Verification items for the finished model (mm, model axes). Face numbers are marked on the shaded views. A direction names the side the tool comes from. Coordinates: 2 decimals unless noted, no trailing zeros. Order: outer loops, then holes, each group sorted by start corner. A loop starts at its lowest first (then second) coordinate and runs counter-clockwise, first axis right, second up. Notation, with made-up numbers: (70.5, 7) -> (78.5, 7) arc R34 cw to (78.5, 42) -> close; hole circle Ø7 at (19, -37.75). An arc over 180 degrees is marked (long way). Answer as CSV lines item,"result".
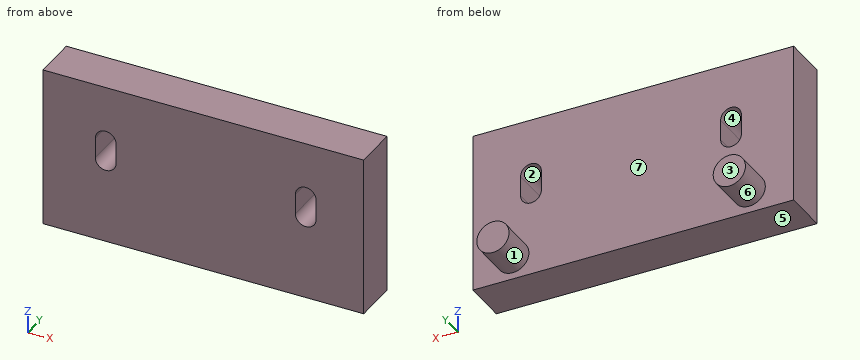
```python
from build123d import *

# Parameters (mm, degrees)
SKETCH1_W           = 301.378206246
SKETCH1_H           = 151.435088782
BOSS_EXTRUDE1_DEPTH = 41.656
CUT_EXTRUDE1_DEPTH  = 214.376
SKETCH3_R           = 15.161110792
BOSS_EXTRUDE2_DEPTH = 35.56


with BuildPart() as part:
    # Sketch1 → Boss-Extrude1 (new body)
    with BuildSketch(Plane(origin=(0, 0, 0), x_dir=(1, 0, 0), z_dir=(0, 1, 0))):
        with Locations((-2.237956977, 0)):
            Rectangle(SKETCH1_W, SKETCH1_H)
    extrude(amount=BOSS_EXTRUDE1_DEPTH)

    # Sketch2 → Cut-Extrude1 (cut)
    with BuildSketch(Plane(origin=(0, 41.656, 0), x_dir=(1, 0, 0), z_dir=(0, 1, 0))):
        with BuildLine():
            Line((-103.753069352, -3.904427399), (-103.753069352, -22.938510969))
            ThreePointArc((-103.753069352, -22.938510969), (-93.992000854, -32.699579467), (-84.230932357, -22.938510969))
            Line((-84.230932357, -22.938510969), (-84.230932357, -3.904427399))
            ThreePointArc((-84.230932357, -3.904427399), (-93.992000854, 5.856641099), (-103.753069352, -3.904427399))
        make_face()
    cut_extrude1 = extrude(amount=-CUT_EXTRUDE1_DEPTH, mode=Mode.SUBTRACT)

    # Sketch3 → Boss-Extrude2 (add)
    with BuildSketch(Plane(origin=(0, 41.656, 0), x_dir=(1, 0, 0), z_dir=(0, 1, 0))):
        with Locations(Location((-111.073870725, 54.487556638, 0), (0, 0, 270))):
            Circle(SKETCH3_R)
    boss_extrude2 = extrude(amount=BOSS_EXTRUDE2_DEPTH)

    # Mirror1: Cut-Extrude1, Boss-Extrude2 across plane
    add(cut_extrude1.mirror(Plane(origin=(0, 0, 0), x_dir=(0, 0, 1), z_dir=(1, 0, 0))), mode=Mode.SUBTRACT)
    add(boss_extrude2.mirror(Plane(origin=(0, 0, 0), x_dir=(0, 0, 1), z_dir=(1, 0, 0))))


solid = part.part
```
Item 1: Section check C-C, the plane x = -118. Record the boundary of the cut face in (y, z), plus the area to 3 significant figures.
Answer list:
outline,"(0, -75.72) -> (41.66, -75.72) -> (41.66, -67.97) -> (77.22, -67.97) -> (77.22, -41) -> (41.66, -41) -> (41.66, 75.72) -> (0, 75.72) -> close"
area,"7,270 mm2"
Item 2: Section check A-A, the plane y = 27. Record the boundary of the cut face in (x, z).
Answer list:
outline,"(-152.93, -75.72) -> (148.45, -75.72) -> (148.45, 75.72) -> (-152.93, 75.72) -> close; hole (-103.75, 3.9) arc R9.76 ccw to (-84.23, 3.9) -> (-84.23, 22.94) arc R9.76 ccw to (-103.75, 22.94) -> close; hole (84.23, 3.9) arc R9.76 ccw to (103.75, 3.9) -> (103.75, 22.94) arc R9.76 ccw to (84.23, 22.94) -> close"
Item 3: Tool access check on the marked faces 1, 2 and 3. Record the directions out of +Z, -Z, +X, -X, +Y, -Y that give a thin tool (end or side, any length) a straight path to the whole face; none if there is none.
Answer list:
face 1,"+Y"
face 2,"+Y, -Y"
face 3,"+Z, -Z, +X, -X, +Y"
Item 4: Section check B-B, the plane y = 60. Record the boundary of the cut face in (x, z).
Answer list:
outline,"circle Ø30.32 at (-111.07, -54.49); circle Ø30.32 at (111.07, -54.49)"
Item 5: Depth check by flat-ended pin: pin 1 Ø6 at (x, y) = (115.5, 55) entering from -Z; pin 2 Ø12 at (x, z) = (2, -36.5) entering from +Y. Enter the tip coordinate at first touch or a pass-through.
Answer list:
pin 1,"z = -69.58"
pin 2,"y = 41.66"
Item 6: Section check D-D, the plane z = 57.5. Record the boundary of the cut face in (x, y).
Answer list:
outline,"(-152.93, 0) -> (148.45, 0) -> (148.45, 41.66) -> (-152.93, 41.66) -> close"
Item 7: Release check for a two-part mould opening along Z. For the marked faces 4, 5, 6 and 7 record: +Z half, -Z half, draft (parallel to the pull), parting line (faces both ways), or undercut.
Answer list:
face 4,"undercut"
face 5,"-Z half"
face 6,"parting line"
face 7,"draft"
Item 8: Thickness scan on line 1 (X direction, y = 37, z = 14); line 2 (Z direction, x = -95, y = 26); line 3 (Y direction, x = -75, z = 12). Record the ranges inside material, lowest first.
Answer list:
line 1,"-152.93 to -103.75, -84.23 to 84.23, 103.75 to 148.45"
line 2,"-75.72 to -5.8, 32.65 to 75.72"
line 3,"0 to 41.66"
